CAD build for the part. Positions are in the model's coordinates, mm. Give positions to 0.01 mm unless a question says otherwise; leave off trailing zeros. Loops run counter-clockwise (first coordinate to the right, second up) from the corner with the lowest first, then second, coordinate; pieces in that order, holes last.
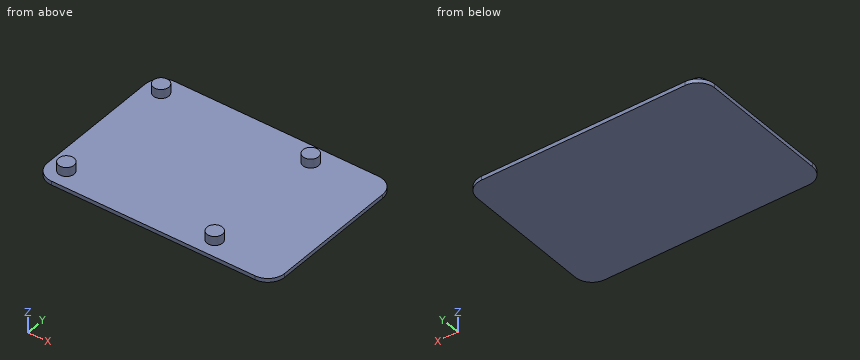
```python
from build123d import *

# Parameters (mm, degrees)
F2_DEPTH = 1.5
F3_R     = 3
F5_DEPTH = 3.5


with BuildPart() as f2:
    # F1 (on Top) → F2 (new body)
    with BuildSketch(Plane.XY):
        with BuildLine():
            Line((39.5, 31.5), (-39.5, 31.5))
            ThreePointArc((-39.5, 31.5), (-44.0961940777, 29.5961940777), (-46, 25))
            Line((-46, 25), (-46, -25))
            ThreePointArc((-46, -25), (-44.0961940777, -29.5961940777), (-39.5, -31.5))
            Line((-39.5, -31.5), (39.5, -31.5))
            ThreePointArc((39.5, -31.5), (44.0961940777, -29.5961940777), (46, -25))
            Line((46, -25), (46, 25))
            ThreePointArc((46, 25), (44.0961940777, 29.5961940777), (39.5, 31.5))
        make_face()
    extrude(amount=F2_DEPTH)

    # F3 (on face) → F5 (join, through all)
    with BuildSketch(Plane.XY.offset(1.5)):
        with Locations((-39.5, 24.5)):
            Circle(F3_R)
        with Locations((18.5, 24.5)):
            Circle(F3_R)
        with Locations((-39, -24.5)):
            Circle(F3_R)
        with Locations((18.5, -24.5)):
            Circle(F3_R)
    extrude(amount=F5_DEPTH)


solid = f2.part
```
1. Saw through at D-D, the plane x = 7. List the corners of the cut face in (y, z), and give its area (3 significant figures).
Responses:
outline: (-31.5, 0) - (31.5, 0) - (31.5, 1.5) - (-31.5, 1.5) - close
area: 94.5 mm2
2. Probe line 1 along Z through (x, y) = (-26.5, 24); line 2 along X through (y, z) = (26, 2.9); line 3 along X through (y, z) = (25.5, 2.05). List the from-to ranges inside material, lowest first.
Responses:
line 1: z = 0 to 1.5
line 2: x = -42.1 to -36.9, 15.9 to 21.1
line 3: x = -42.33 to -36.67, 15.67 to 21.33
3. Drop flat-ended pins along their axis: pin 1 (1 mm diameter, centred on x = -8, y = 15.5, fed in from +Z); pin 2 (4 mm diameter, centred on x = -1, y = -6.5, fed in from -Z); pin 3 (1 mm diameter, centred on x = 16.5, z = 3, fed in from -Y). Give the stop position or say it passes through.
Responses:
pin 1: stops at z = 1.5
pin 2: stops at z = 0
pin 3: stops at y = -27.1
4. Saw through at B-B, the plane z = 3.35. List the corners of the cut face in (x, y).
Responses:
outline: circle Ø6 at (-39.5, 24.5); circle Ø6 at (-39, -24.5); circle Ø6 at (18.5, -24.5); circle Ø6 at (18.5, 24.5)
5. Saw through at A-A, the plane x = 18.5. List the corners of the cut face in (y, z), and give its area (4 significant figures).
Responses:
outline: (-31.5, 0) - (31.5, 0) - (31.5, 1.5) - (27.5, 1.5) - (27.5, 5) - (21.5, 5) - (21.5, 1.5) - (-21.5, 1.5) - (-21.5, 5) - (-27.5, 5) - (-27.5, 1.5) - (-31.5, 1.5) - close
area: 136.5 mm2
6. Saw through at C-C, the plane y = -23. List the corners of the cut face in (x, z).
Responses:
outline: (-46, 0) - (46, 0) - (46, 1.5) - (21.1, 1.5) - (21.1, 5) - (15.9, 5) - (15.9, 1.5) - (-36.4, 1.5) - (-36.4, 5) - (-41.6, 5) - (-41.6, 1.5) - (-46, 1.5) - close
